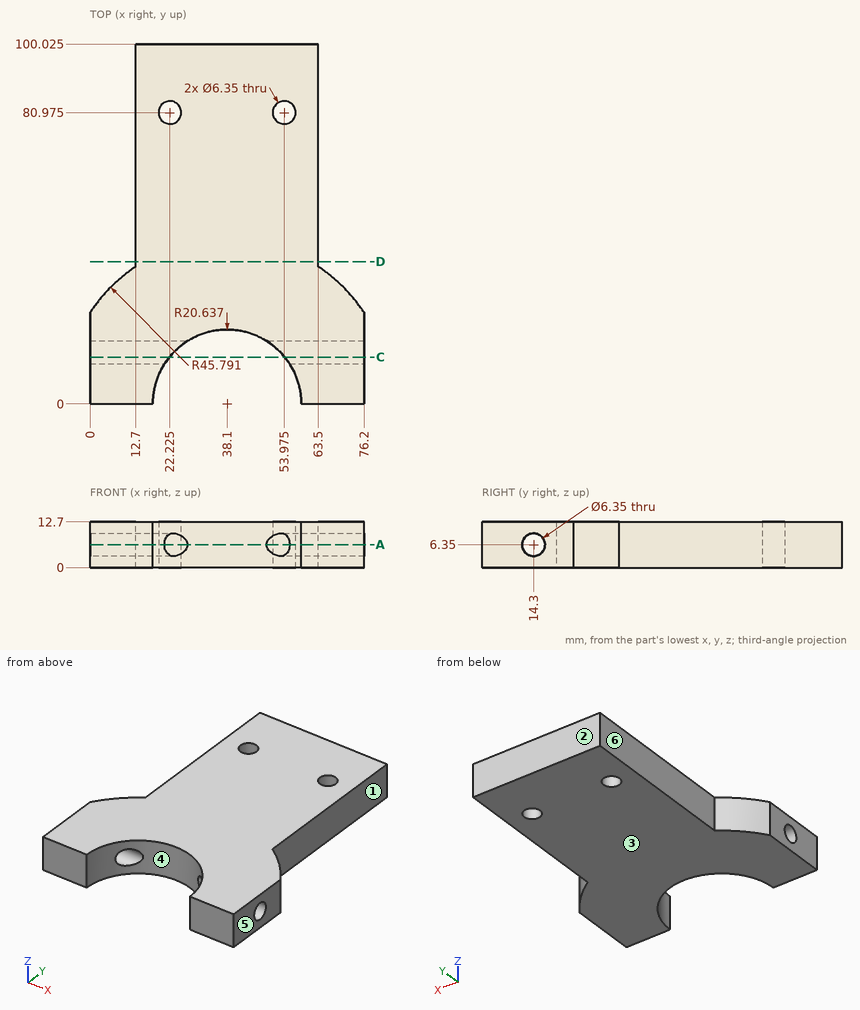
Part print with two shaded views. Sizes in mm from the minimum x, y, z corner. A direction names the side the tool comes from. Coordinates: 2 decimals unless noted, no trailing zeros. Loops run counter-clockwise (first coordinate to the right, second up) from the corner with the lowest first, then second, coordinate; pieces in that order, holes last. Notation, with made-up numbers: M 25.5,63.5 L 82.5,63.5 A28 cw 82.5,95.5 Z; hole C 4,55 d6. An arc over 180 degrees is marked long. Use CSV: the item, a comma, the result in double quotes. Start each with the question number.
1. Flat gauge pins, fed straight in: pin 1 (4 mm diameter, centred on y = 38, z = 4.5, fed in from -X); pin 2 (4 mm diameter, centred on y = 14.3, z = 6.35, fed in from -X); pin 3 (3 mm diameter, centred on y = 88, z = 6, fed in from -X); pin 4 (1.5 mm diameter, centred on x = 64.5, z = 11, fed in from +Y). Where does each tip first touch, or does it go through?
2. Band-saw the part on C-C, the plane y = 13. List the corners of the cut face in (x, z).
3. Band-saw the part on D-D, the plane y = 39.5. List the corners of the cut face in (x, z), then the cut area to 3 significant figures.
4. Two-plate mould, pull along X, no slides. Class the marked faces 3, 4, 5 and 6: pulls with the +X half, pulls with the -X half, needs draft (parallel to the pull), parting line crosses it, or undercut.
5. Probe probe 1 along X at (y, z) = (71, 10.5); probe 2 along Y at (x, z) = (73, 4.25) (1 decimal); probe 3 along Y at (x, z) = (61.5, 4.75) (1 decimal). List the from-to ranges inside material, lowest first. Write a range as [from, to].
6. Band-saw the part on A-A, the plane z = 6.35. Give the number of separate pieces and of enclosed holes in the cut face, then the cut area to 3 significant figures.
7. Tool access for the marked faces 1 and 2: list every direction of +Z, -Z, +X, -X, +Y, -Y with a clear straight run to the whole face (end or side of a thin tool).
Entries:
1,pin 1,"stops at x = 9.8"
1,pin 2,"passes through"
1,pin 3,"stops at x = 12.7"
1,pin 4,"stops at y = 37.93"
2,outline,"M 0,0 L 22.07,0 L 22.07,3.45 L 0,3.45 Z; M 0,9.25 L 22.07,9.25 L 22.07,12.7 L 0,12.7 Z; M 54.13,0 L 76.2,0 L 76.2,3.45 L 54.13,3.45 Z; M 54.13,9.25 L 76.2,9.25 L 76.2,12.7 L 54.13,12.7 Z"
3,outline,"M 12.7,0 L 63.5,0 L 63.5,12.7 L 12.7,12.7 Z"
3,area,"645 mm2"
4,face 3,"needs draft"
4,face 4,"undercut"
4,face 5,"pulls with the +X half"
4,face 6,"pulls with the -X half"
5,probe 1,"x = [12.7, 63.5]"
5,probe 2,"y = [0, 11.9], [16.7, 29.6]"
5,probe 3,"y = [0, 11.6], [17, 100]"
6,separate pieces,"3"
6,enclosed holes,"2"
6,area,"4,880 mm2"
7,face 1,"+Z, -Z, +X, +Y"
7,face 2,"+Z, -Z, +X, -X, +Y"
